Part model, mm, in its own coordinate system. A direction names the side the tool comes from. Coordinates: 2 decimals unless noted, no trailing zeros. Order: outer loops, then holes, each group sorted by start corner. A loop starts at its lowest first (then second) coordinate and runs counter-clockwise, first axis right, second up.
from build123d import *

# Parameters (mm, degrees)
ESBO_O1_W                = 160
ESBO_O1_H                = 70
RESSALTO_EXTRUS_O1_DEPTH = 10
FURO_COM_FOLGA_DE_M33_D  = 3.4
ESBO_O6_R                = 5
CORTE_EXTRUS_O1_DEPTH    = 10
FURO_COM_FOLGA_DE_M61_D  = 6.6


with BuildPart() as part:
    # Esboço1 → Ressalto-extrusão1 (new body)
    with BuildSketch(Plane(origin=(0, 0, 92.2731107), x_dir=(-1, 0, 0), z_dir=(0, 0, -1))):
        with Locations((66.819307324, 485.108658775)):
            Rectangle(ESBO_O1_W, ESBO_O1_H)
    extrude(amount=RESSALTO_EXTRUS_O1_DEPTH)

    # Furo com folga de M33 (through all)
    with Locations(Plane.XY.offset(92.2731107)):
        with Locations((-106.819307324, 515.108658775), (-26.819307324, 515.108658775), (-26.819307324, 455.108658775), (-106.819307324, 455.108658775)):
            Hole(FURO_COM_FOLGA_DE_M33_D / 2)

    # Esboço6 → Corte-extrusão1 (cut)
    with BuildSketch(Plane.XY.offset(93.7731107)):
        with Locations((-34.419307324, 480.308658775)):
            Circle(ESBO_O6_R)
        with Locations((-99.219307324, 494.708658775)):
            Circle(ESBO_O6_R)
    extrude(amount=-CORTE_EXTRUS_O1_DEPTH, mode=Mode.SUBTRACT)

    # Furo com folga de M61 (through all)
    with Locations(Plane.XY.offset(83.7731107)):
        with Locations((-99.219307324, 494.708658775), (-34.419307324, 480.308658775)):
            Hole(FURO_COM_FOLGA_DE_M61_D / 2)


solid = part.part
Q1. Which spindle directions (+Z, -Z, +X, -X, +Y, -Y) get a long thin tool onto all of the face, cutting with end or side? Do faces 5 (the face through (-33, 477, 83.773)), 6 (the face through (13.181, 485, 87)). Say none if no direction does.
Results list:
face 5: +Z
face 6: +Z, -Z, +X, +Y, -Y
Q2. Wall check: line 1 along X through (y, z) = (455, 87); line 2 along X through (y, z) = (456, 86); line 3 along Y through (x, z) = (-103, 87.75). Give the ranges that are in metal, low to high.
Results list:
line 1: x = -146.82 to -108.52, -105.12 to -28.52, -25.12 to 13.18
line 2: x = -146.82 to -108.27, -105.37 to -28.27, -25.37 to 13.18
line 3: y = 450.11 to 491.44, 497.98 to 520.11
Q3. Pin check, flat tips, straight feed: pin 1 Ø3 at (x, y) = (-26.82, 515.11) entering from -Z; pin 2 Ø3 at (x, y) = (-97, 497) entering from +Z. Stop position of each tip, or through.
Results list:
pin 1: passes through
pin 2: stops at z = 83.77
Q4. Mould opens along Y. For faces 1 (the face through (-35.94, 477.38, 83.01)), 2 (the face through (-66, 450.109, 87)), 3 (the face through (-66, 520.109, 87)), 4 (the face through (-66, 486, 82.273)) say: pulls with the +Y half, pulls with the -Y half, needs draft (parallel to the pull), parting line crosses it, or undercut.
Results list:
face 1: undercut
face 2: pulls with the -Y half
face 3: pulls with the +Y half
face 4: needs draft
Q5. Cut at A-A on z = 88.5. Write the cut outline in (x, y), and give its area (3 significant figures).
Results list:
outline: (-146.82, 450.11) - (13.18, 450.11) - (13.18, 520.11) - (-146.82, 520.11) - close; hole circle Ø3.4 at (-106.82, 455.11); hole circle Ø3.4 at (-106.82, 515.11); hole circle Ø10 at (-99.22, 494.71); hole circle Ø10 at (-34.42, 480.31); hole circle Ø3.4 at (-26.82, 455.11); hole circle Ø3.4 at (-26.82, 515.11)
area: 11,000 mm2
